Work out the finished part from the listing and answer in its coordinate system (mm). A direction names the side the tool comes from. Round coordinates to 2 decimals unless told otherwise and drop trailing zeros. Loops run counter-clockwise (first coordinate to the right, second up) from the corner with the lowest first, then second, coordinate; pieces in that order, holes last. Notation, with made-up numbers: (83, 54.5) - (132, 54.5) arc R20 ccw to (132, 59.5) - close; hole circle Ø4 at (-15.5, -27.5). An arc over 180 degrees is marked (long way). Use CSV: the item, a comma, the result in double quotes. Start each with the question number.
from build123d import *

# Parameters (mm, degrees)
SKETCH1_W                      = 114.3
SKETCH1_H                      = 63.5
BASE_FLANGE1_DEPTH             = 2.032
EDGE_FLANGE1_STRIP_W           = 14.478
EDGE_FLANGE1_STRIP_H           = 2.032
EDGE_FLANGE1_STRIP_CUT_DEPTH   = 114.3
EDGE_FLANGE1_STRIP_2_W         = 14.478
EDGE_FLANGE1_STRIP_2_H         = 2.032
EDGE_FLANGE1_STRIP_CUT_2_DEPTH = 114.3
EDGE_FLANGE1_DEPTH             = 114.3
EDGE_FLANGE1_BEND_DEPTH        = 114.3
EDGE_FLANGE2_DEPTH             = 63.5
EDGE_FLANGE2_2_DEPTH           = 5.207
EDGE_FLANGE2_START             = 58.293
EDGE_FLANGE2_3_DEPTH           = 5.207
EDGE_FLANGE2_START_2           = 5.207
EDGE_FLANGE2_4_DEPTH           = 53.086


# Read off the part's stored shape, not the designer's step: Edge-Flange2
# Sheet-metal steps are written as plain solids
with BuildPart() as part:
    # Sketch1 → Base-Flange1 (new body)
    with BuildSketch(Plane(origin=(0, 0, 0), x_dir=(0, 0, -1), z_dir=(1, 0, 0))):
        with Locations((57.15, 31.75)):
            Rectangle(SKETCH1_W, SKETCH1_H)
    extrude(amount=-BASE_FLANGE1_DEPTH)

    # Edge-Flange1 strip (across the edge) → Edge-Flange1 strip cut (cut)
    with BuildSketch(Plane(origin=(0, 63.5, -114.3), x_dir=(0, -1, 0), z_dir=(0, 0, 1))):
        with Locations((-2.032, -1.016)):
            Rectangle(EDGE_FLANGE1_STRIP_W, EDGE_FLANGE1_STRIP_H)
    extrude(amount=EDGE_FLANGE1_STRIP_CUT_DEPTH, mode=Mode.SUBTRACT)

    # Edge-Flange1 strip 2 (across the edge) → Edge-Flange1 strip cut 2 (cut)
    with BuildSketch(Plane.YX):
        with Locations((-2.032, -1.016)):
            Rectangle(EDGE_FLANGE1_STRIP_2_W, EDGE_FLANGE1_STRIP_2_H)
    extrude(amount=EDGE_FLANGE1_STRIP_CUT_2_DEPTH, mode=Mode.SUBTRACT)

    # Edge-Flange1 section (across the edge) → Edge-Flange1 (add)
    with BuildSketch(Plane(origin=(0, 63.5, -114.3), x_dir=(0, -1, 0), z_dir=(0, 0, 1))):
        with BuildLine():
            Line((0, 3.175), (0, 29.718))
            Line((0, 29.718), (2.032, 29.718))
            Line((2.032, 29.718), (2.032, 3.175))
            ThreePointArc((2.032, 3.175), (2.96193597, 0.92993597), (5.207, 0))
            Line((5.207, 0), (5.207, -2.032))
            ThreePointArc((5.207, -2.032), (1.52509499, -0.50690501), (0, 3.175))
        make_face()
    extrude(amount=EDGE_FLANGE1_DEPTH)

    # Edge-Flange1 section 2 (across the edge) → Edge-Flange1 bend (add)
    with BuildSketch(Plane.YX):
        with BuildLine():
            Line((0, 3.175), (0, 29.718))
            Line((0, 29.718), (2.032, 29.718))
            Line((2.032, 29.718), (2.032, 3.175))
            ThreePointArc((2.032, 3.175), (2.96193597, 0.92993597), (5.207, 0))
            Line((5.207, 0), (5.207, -2.032))
            ThreePointArc((5.207, -2.032), (1.52509499, -0.50690501), (0, 3.175))
        make_face()
    extrude(amount=EDGE_FLANGE1_BEND_DEPTH)

    # Edge-Flange2 outline → Edge-Flange2 (cut)
    with BuildSketch(Plane(origin=(0, 0, 0), x_dir=(1, 0, 0), z_dir=(0, 1, 0))):
        with BuildLine():
            Line((3.175, 0), (3.175, 3.175))
            Line((3.175, 3.175), (0, 3.175))
            ThreePointArc((0, 3.175), (0.92993597, 0.92993597), (3.175, 0))
        make_face()
        with BuildLine():
            ThreePointArc((-0.95201151, 0), (-1.754614485, 1.498172628), (-2.032, 3.175))
            Line((-2.032, 3.175), (-2.032, 0))
            Line((-2.032, 0), (-0.95201151, 0))
        make_face()
    extrude(amount=EDGE_FLANGE2_DEPTH, mode=Mode.SUBTRACT)

    # Edge-Flange2 2 outline → Edge-Flange2 2 (cut)
    with BuildSketch(Plane(origin=(0, 0, 0), x_dir=(1, 0, 0), z_dir=(0, 1, 0))):
        with BuildLine():
            ThreePointArc((3.175, 0), (0.92993597, 0.92993597), (0, 3.175))
            Line((0, 3.175), (-2.032, 3.175))
            ThreePointArc((-2.032, 3.175), (-1.754614485, 1.498172628), (-0.95201151, 0))
            Line((-0.95201151, 0), (3.175, 0))
        make_face()
    extrude(amount=EDGE_FLANGE2_2_DEPTH, mode=Mode.SUBTRACT)

    # Edge-Flange2 3 outline → Edge-Flange2 3 (cut)
    with BuildSketch(Plane(origin=(0, 0, 0), x_dir=(1, 0, 0), z_dir=(0, 1, 0)).offset(EDGE_FLANGE2_START)):
        with BuildLine():
            ThreePointArc((3.175, 0), (0.92993597, 0.92993597), (0, 3.175))
            Line((0, 3.175), (-2.032, 3.175))
            ThreePointArc((-2.032, 3.175), (-1.754614485, 1.498172628), (-0.95201151, 0))
            Line((-0.95201151, 0), (3.175, 0))
        make_face()
    extrude(amount=EDGE_FLANGE2_3_DEPTH, mode=Mode.SUBTRACT)

    # Edge-Flange2 4 outline → Edge-Flange2 4 (add)
    with BuildSketch(Plane(origin=(0, 0, 0), x_dir=(1, 0, 0), z_dir=(0, 1, 0)).offset(EDGE_FLANGE2_START_2)):
        with BuildLine():
            Line((0, 3.175), (0, 0))
            Line((0, 0), (-0.95201151, 0))
            ThreePointArc((-0.95201151, 0), (0.874932175, -1.496459836), (3.175, -2.032))
            Line((3.175, -2.032), (29.718, -2.032))
            Line((29.718, -2.032), (29.718, 0))
            Line((29.718, 0), (3.175, 0))
            ThreePointArc((3.175, 0), (0.92993597, 0.92993597), (0, 3.175))
        make_face()
    extrude(amount=EDGE_FLANGE2_4_DEPTH)


solid = part.part
Item 1: A cutting plane is placed at A-A (z = -46). Determine the outline of the cut face in (x, y) (3 decimals), plus the area to 3 significant figures.
Item 2: A cutting plane is placed at C-C (y = 12.5). Determine the outline of the cut face in (x, z) (3 decimals), plus the area to 3 significant figures.
Item 3: Find the intervals of material crossed by probe 1 along Y at (x, z) = (21, -11.5); probe 2 along Z at (x, y) = (7, 12.5); probe 3 along X at (y, z) = (26.5, -40), in increasing order. Write a range as [from, to].
Item 4: A cutting plane is placed at D-D (x = 2). Determine the outline of the cut face in (y, z) (3 decimals), plus the area to 3 significant figures.
Item 5: Each of these flat-tipped pins is pushed along its axis until it touches: pin 1 Ø1.6 at (x, y) = (21, 0.5) entering from +Z; pin 2 Ø10 at (y, z) = (8.5, -64.5) entering from +X; pin 3 Ø2 at (x, y) = (19, 47.5) entering from -Z; pin 4 Ø1.6 at (x, z) = (19.5, -0.5) entering from -Y. Where does it stop, or does it pass through?
Item 6: Which of the six approach directions +Z, -Z, +X, -X, +Y, -Y give full straight-line access (tool end or side, diameter ignored) to faces 1 (the flat face through (17, 31, 0)), 2 (the flat face through (14, 58.293, 1)), 3 (the cylindrical face through (0.95, 60.56, -59.52)), 4 (the flat face through (1, 61, -3.175)), 5 (the flat face through (14, 5.207, 1))?
Item 7: The mould has two halves that part along Y. Classify faces 6 (the flat face through (17, 2.032, -56)), 7 (the flat face through (0.6, 2.6, -3.175)), 8 (the flat face through (16, 0, -56)): pulls with the +Y half, pulls with the -Y half, needs draft (parallel to the pull), parting line crosses it, or undercut.
Item 8: A cutting plane is placed at B-B (x = 23). Determine the outline of the cut face in (y, z), plus the area to 3 significant figures.
Result sheet:
1,outline,"(-2.032, 5.207) arc R5.207 ccw to (3.175, 0) - (29.718, 0) - (29.718, 2.032) - (3.175, 2.032) arc R3.175 cw to (0, 5.207) - (0, 58.293) arc R3.175 cw to (3.175, 61.468) - (29.718, 61.468) - (29.718, 63.5) - (3.175, 63.5) arc R5.207 ccw to (-2.032, 58.293) - close"
1,area,"242 mm^2"
2,outline,"(-2.032, -114.3) - (0, -114.3) - (0, -3.175) arc R3.175 cw to (3.175, 0) - (29.718, 0) - (29.718, 2.032) - (3.175, 2.032) arc R5.207 ccw to (-2.032, -3.175) - close"
2,area,"293 mm^2"
3,probe 1,"[0, 2.03], [61.47, 63.5]"
3,probe 2,"[0, 2.03]"
3,probe 3,"[-2.03, 0]"
4,outline,"(0.134, -114.3) - (2.257, -114.3) - (2.257, -3.175) - (0.134, -3.175) - close; (5.207, -0.225) - (58.293, -0.225) - (58.293, 1.898) - (5.207, 1.898) - close; (61.243, -114.3) - (63.366, -114.3) - (63.366, -3.175) - (61.243, -3.175) - close"
4,area,"585 mm^2"
5,pin 1,"z = 0"
5,pin 2,"x = 0.5"
5,pin 3,"z = 0"
5,pin 4,"y = 0"
6,face 1,"-Z, +X"
6,face 2,"+Z, +X, -X, +Y"
6,face 3,"+Z, -Z, +X"
6,face 4,"+Z, -X, +Y"
6,face 5,"+Z, +X, -X, -Y"
7,face 6,"undercut"
7,face 7,"needs draft"
7,face 8,"pulls with the -Y half"
8,outline,"(0, -114.3) - (2.03, -114.3) - (2.03, 0) - (0, 0) - close; (5.21, 0) - (58.29, 0) - (58.29, 2.03) - (5.21, 2.03) - close; (61.47, -114.3) - (63.5, -114.3) - (63.5, 0) - (61.47, 0) - close"
8,area,"572 mm^2"
